For this review, take the finished solid that the model builds, in its own axes (mm). Face numbers are marked on the shaded views. Give positions to 0.01 mm unless a question says otherwise; leave off trailing zeros. Order: outer loops, then holes, each group sorted by start corner. A loop starts at its lowest first (then second) coordinate and runs counter-clockwise, first axis right, second up. Notation, with made-up numbers: (-31.75, 82.5) -> (19.25, 82.5) arc R28 ccw to (19.25, 100.5) -> close; hole circle Ø11 at (73.5, -3). An arc over 180 degrees is marked (long way). Return JSON: item names as keys, results as strings. Group by question number.
1) Add section C-C (z = 4.5). Give the boundary of the cut face in (x, y), then the cut area to 3 significant figures.
2) Add section A-A (x = 0). Give the boundary of the cut face in (y, z).
3) The part is to be moulded in two halves that separate along X. For the marked faces 1, 2 and 3, say which applies: released by +X, released by -X, zero draft, split by the parting line, or undercut.
4) To check wall thickness, follow line 1 along Y through (x, z) = (0, 3); line 2 along Y through (x, z) = (5, 3); line 3 along Z through (x, y) = (-4, 6.5). State the ranges of each line that lie inside material, in increasing order.
5) Insertion check: P1, Ø3, axis at x = -3.5, z = 3.5, coming from the -Y side; P2, Ø3, axis at y = 4.5, z = 3.5, coming from the -X side; P3, Ø1.5, axis at x = -4, z = 5, coming from the +Y side. Each pin has a flat end and moves straight along its axis. Give the tip position at first contact, or say it passes through.
from build123d import *

# Parameters (mm, degrees)
F0_R     = 10
F0_R_2   = 7.5
F1_DEPTH = 1.5
F0_R_3   = 6.1
F2_DEPTH = 8
F4_R     = 1


# Not quite as in the source:
# - a fillet or chamfer that OpenCascade refuses, or shapes differently, is made with other operations: its cross-section is extruded or revolved along the edge and cut away or added


with BuildPart() as f1:
    # F0 (on Top) → F1 (new body)
    with BuildSketch(Plane.XY):
        Circle(F0_R)
        Circle(F0_R_2, mode=Mode.SUBTRACT)
    extrude(amount=F1_DEPTH)

    # F0 (on Top) → F2 (join)
    with BuildSketch(Plane.XY):
        Circle(F0_R_2)
        Circle(F0_R_3, mode=Mode.SUBTRACT)
    extrude(amount=F2_DEPTH)

    # F3: fillet of radius 2 on 1 edges, made by hand

    # F3_s1 → F3_t2 (revolve, cut)
    with BuildSketch(Plane.XZ):
        with BuildLine():
            ThreePointArc((10, 1.5), (9.2882531983, 0.4188611699), (8.0635083269, 0))
            Line((8.0635083269, 0), (10, 0))
            Line((10, 0), (10, 1.5))
        make_face()
    revolve(axis=Axis((0, 0, 0), (0, 0, 1)), mode=Mode.SUBTRACT)

    # F4
    f4_edges = [f1.edges().sort_by_distance(p)[0] for p in [
        (-6.1, 0, 8),
    ]]
    fillet(f4_edges, radius=F4_R)


solid = f1.part
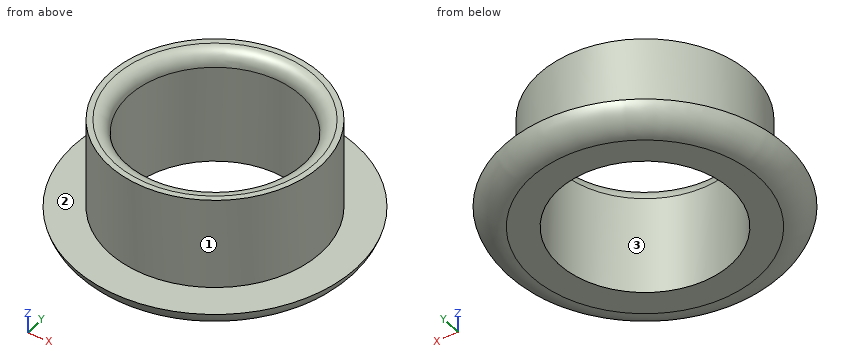
Evaluation:
{
 "1": {"outline": "circle Ø15 at (0, 0); hole circle Ø12.2 at (0, 0)", "area": "59.8 mm^2"},
 "2": {"outline": "(-10, 1.5) arc R2 ccw to (-8.06, 0) -> (-6.1, 0) -> (-6.1, 7) arc R1 ccw to (-7.1, 8) -> (-7.5, 8) -> (-7.5, 1.5) -> close; (6.1, 0) -> (8.06, 0) arc R2 ccw to (10, 1.5) -> (7.5, 1.5) -> (7.5, 8) -> (7.1, 8) arc R1 ccw to (6.1, 7) -> close"},
 "3": {"face 1": "split by the parting line", "face 2": "zero draft", "face 3": "undercut"},
 "4": {"line 1": "-7.5 to -6.1, 6.1 to 7.5", "line 2": "-5.59 to -3.49, 3.49 to 5.59", "line 3": "0 to 1.5"},
 "5": {"P1": "y = -7.23", "P2": "x = -6.87", "P3": "y = 6.76"}
}
